Source: CAD feature listing. Evaluate the final solid. Frame: model axes, mm. A direction names the side the tool comes from. Give positions to 0.01 mm unless a question says otherwise; leave off trailing zeros. Loops run counter-clockwise (first coordinate to the right, second up) from the corner with the lowest first, then second, coordinate; pieces in that order, holes last.
from build123d import *

# Parameters (mm, degrees)
SKETCH1_W                   = 65
SKETCH1_H                   = 70
BOSS_EXTRUDE1_DEPTH         = 8
FILLET1_R                   = 5
SKETCH2_W                   = 41
SKETCH2_H                   = 4
BOSS_EXTRUDE2_DEPTH         = 7.87989528
FILLET2_R                   = 2
SKETCH_1_R                  = 1.75
CUT_EXTRUDE_1_DEPTH         = 71
HOLE_WIZARD_M3_1_D          = 2.5
HOLE_WIZARD_M3_1_DEPTH      = 10
HOLE_WIZARD_M3_1_TIP        = 0.751075774
SKETCH_11_W                 = 65
SKETCH_11_H                 = 70.4
EXTRUDE_1_DEPTH             = 2.9
FILLET_2_R                  = 5
FILLET_3_R                  = 5
FILLET_4_R                  = 5
FILLET_5_R                  = 5
SKETCH_24_W                 = 1.25
SKETCH_24_H                 = 2.901
HOLE_WIZARD_M3_2_AT_2_COUNT = 2
HOLE_WIZARD_M3_2_AT_2_PITCH = 50
HOLE_WIZARD_M3_2_AT_3_COUNT = 2
HOLE_WIZARD_M3_2_AT_3_PITCH = 50
HOLE_WIZARD_M3_2_AT_4_COUNT = 2
HOLE_WIZARD_M3_2_AT_4_PITCH = 70.710678119
HOLE_WIZARD_M4_2_AT_2_COUNT = 2
HOLE_WIZARD_M4_2_AT_2_PITCH = 17.145
HOLE_WIZARD_M4_2_AT_3_COUNT = 2
HOLE_WIZARD_M4_2_AT_3_PITCH = 34.29
HOLE_WIZARD_M4_2_AT_4_COUNT = 2
HOLE_WIZARD_M4_2_AT_4_PITCH = 29.696011096
SKETCH_28_W                 = 16.34592277
SKETCH_28_H                 = 84.825432557
CUT_EXTRUDE_4_DEPTH         = 66
HOLE_WIZARD_M6_1_D          = 5


with BuildPart() as part:
    # Sketch1 → Boss-Extrude1 (new body)
    with BuildSketch(Plane.XY):
        Rectangle(SKETCH1_W, SKETCH1_H)
    extrude(amount=BOSS_EXTRUDE1_DEPTH)

    # Fillet1
    fillet1_edges = [part.edges().sort_by_distance(p)[0] for p in [
        (32.5, -35, 4),
        (-32.5, -35, 4),
        (-32.5, 35, 4),
        (32.5, 35, 4),
    ]]
    fillet(fillet1_edges, radius=FILLET1_R)

    # Sketch2 → Boss-Extrude2 (add)
    with BuildSketch(Plane.XY.offset(8)):
        with Locations((0, -33)):
            Rectangle(SKETCH2_W, SKETCH2_H)
    extrude(amount=BOSS_EXTRUDE2_DEPTH)

    # Fillet2
    fillet2_edges = [part.edges().sort_by_distance(p)[0] for p in [
        (-20.5, -33, 8),
        (20.5, -33, 8),
        (-20.5, -33, 15.87989528),
        (20.5, -33, 15.87989528),
    ]]
    fillet(fillet2_edges, radius=FILLET2_R)

    # 草图1 → 切除-拉伸1 (cut, through all)
    with BuildSketch(Plane.XZ.offset(35)):
        with Locations((-16, 11.87989528)):
            Circle(SKETCH_1_R)
        with Locations((0, 11.87989528)):
            Circle(SKETCH_1_R)
        with Locations((16, 11.87989528)):
            Circle(SKETCH_1_R)
    extrude(amount=-CUT_EXTRUDE_1_DEPTH, mode=Mode.SUBTRACT)

    # M3 螺纹孔1
    with Locations(Plane(origin=(25, -19, 0), x_dir=(-1, 0, 0), z_dir=(0, 0, -1))):
        with Locations((0, 0), (0, 50), (50, 50), (50, 0)):
            Hole(HOLE_WIZARD_M3_1_D / 2, depth=HOLE_WIZARD_M3_1_DEPTH)
            with Locations((0, 0, -(HOLE_WIZARD_M3_1_DEPTH + HOLE_WIZARD_M3_1_TIP / 2))):  # 118° drill point
                Cone(0, HOLE_WIZARD_M3_1_D / 2, HOLE_WIZARD_M3_1_TIP, mode=Mode.SUBTRACT)

    # M6 螺纹孔1 (through all)
    with Locations(Plane(origin=(12.3825, 6, 0), x_dir=(-1, 0, 0), z_dir=(0, 0, -1))):
        with Locations((0, 0), (24.765, 0)):
            Hole(HOLE_WIZARD_M6_1_D / 2)


with BuildPart() as body_2:
    # 草图11 → 凸台-拉伸1 (new body)
    with BuildSketch(Plane(origin=(0, 0, -30.31), x_dir=(-1, 0, 0), z_dir=(0, 0, -1))):
        with Locations((0, 0.2)):
            Rectangle(SKETCH_11_W, SKETCH_11_H)
    extrude(amount=-EXTRUDE_1_DEPTH)

    # 圆角2
    fillet_2_edges = [body_2.edges().sort_by_distance(p)[0] for p in [
        (-32.5, 35.4, -28.86),
    ]]
    fillet(fillet_2_edges, radius=FILLET_2_R)

    # 圆角3
    fillet_3_edges = [body_2.edges().sort_by_distance(p)[0] for p in [
        (-32.5, -35, -28.86),
    ]]
    fillet(fillet_3_edges, radius=FILLET_3_R)

    # 圆角4
    fillet_4_edges = [body_2.edges().sort_by_distance(p)[0] for p in [
        (32.5, -35, -28.86),
    ]]
    fillet(fillet_4_edges, radius=FILLET_4_R)

    # 圆角5
    fillet_5_edges = [body_2.edges().sort_by_distance(p)[0] for p in [
        (32.5, 35.4, -28.86),
    ]]
    fillet(fillet_5_edges, radius=FILLET_5_R)

    # 草图24 → M3 螺纹孔2 (revolve, cut)
    with BuildSketch(Plane(origin=(25, 31, -30.31), x_dir=(0, 1, 0), z_dir=(1, 0, 0))):
        with Locations((0.625, 1.4505)):
            Rectangle(SKETCH_24_W, SKETCH_24_H)
    hole_wizard_m3_2 = revolve(axis=Axis((25, 31, -36.66), (0, 0, 1)), mode=Mode.SUBTRACT)

    # M3 螺纹孔2 at 2: M3 螺纹孔2 ×2
    with Locations(*[(-i * HOLE_WIZARD_M3_2_AT_2_PITCH, 0, 0) for i in range(1, HOLE_WIZARD_M3_2_AT_2_COUNT)]):
        add(hole_wizard_m3_2, mode=Mode.SUBTRACT)

    # M3 螺纹孔2 at 3: M3 螺纹孔2 ×2
    with Locations(*[(0, -i * HOLE_WIZARD_M3_2_AT_3_PITCH, 0) for i in range(1, HOLE_WIZARD_M3_2_AT_3_COUNT)]):
        add(hole_wizard_m3_2, mode=Mode.SUBTRACT)

    # M3 螺纹孔2 at 4: M3 螺纹孔2 ×2
    with Locations(*[Vector(-0.707106781, -0.707106781, 0) * (i * HOLE_WIZARD_M3_2_AT_4_PITCH) for i in range(1, HOLE_WIZARD_M3_2_AT_4_COUNT)]):
        add(hole_wizard_m3_2, mode=Mode.SUBTRACT)

    # 草图27 → M4 六角凹头螺钉的柱形沉头孔2 (revolve, cut)
    with BuildSketch(Plane(origin=(9.41775, -9.820005548, -30.31), x_dir=(0, 1, 0), z_dir=(1, 0, 0))):
        Polygon((0, 0), (0, 38.31), (2.25, 38.31), (2.25, 1.5), (4, 1.5), (4, 0), align=None)
    hole_wizard_m4_2 = revolve(axis=Axis((9.41775, -9.820005548, -36.66), (0, 0, 1)), mode=Mode.SUBTRACT)

    # M4 六角凹头螺钉的柱形沉头孔2 at 2: M4 六角凹头螺钉的柱形沉头孔2 ×2
    with Locations(*[(-i * HOLE_WIZARD_M4_2_AT_2_PITCH, 0, 0) for i in range(1, HOLE_WIZARD_M4_2_AT_2_COUNT)]):
        add(hole_wizard_m4_2, mode=Mode.SUBTRACT)

    # M4 六角凹头螺钉的柱形沉头孔2 at 3: M4 六角凹头螺钉的柱形沉头孔2 ×2
    with Locations(*[Vector(-0.5, 0.866025404, 0) * (i * HOLE_WIZARD_M4_2_AT_3_PITCH) for i in range(1, HOLE_WIZARD_M4_2_AT_3_COUNT)]):
        add(hole_wizard_m4_2, mode=Mode.SUBTRACT)

    # M4 六角凹头螺钉的柱形沉头孔2 at 4: M4 六角凹头螺钉的柱形沉头孔2 ×2
    with Locations(*[(0, i * HOLE_WIZARD_M4_2_AT_4_PITCH, 0) for i in range(1, HOLE_WIZARD_M4_2_AT_4_COUNT)]):
        add(hole_wizard_m4_2, mode=Mode.SUBTRACT)

    # 草图28 → 切除-拉伸4 (cut, through all)
    with BuildSketch(Plane(origin=(32.5, 0, 0), x_dir=(0, 0, -1), z_dir=(1, 0, 0))):
        with Locations((29.455626585, -1.857491224)):
            Rectangle(SKETCH_28_W, SKETCH_28_H)
    extrude(amount=-CUT_EXTRUDE_4_DEPTH, mode=Mode.SUBTRACT)


solid = part.part
1) Ray query, probe 1 along X at (y, z) = (5.5, 3); probe 2 along Y at (x, z) = (25, 2); probe 3 along Y at (x, z) = (13.5, 14). Return the intervals inside material, ascending.
Checks:
probe 1: x = -32.5 to -14.83, -9.93 to 9.93, 14.83 to 32.5
probe 2: y = -35 to -20.25, -17.75 to 29.75, 32.25 to 35
probe 3: y = -35 to -31
2) Cut plane C-C (x = 16). Return loops of the section in (y, z).
Checks:
outline: (-35, 0) - (35, 0) - (35, 8) - (-31, 8) - (-31, 10.13) - (-35, 10.13) - close; (-35, 13.63) - (-31, 13.63) - (-31, 15.88) - (-35, 15.88) - close
3) Cut plane D-D (z = 1.5). Return loops of the section in (x, y), and give its area (3 significant figures).
Checks:
outline: (-32.5, -30) arc R5 ccw to (-27.5, -35) - (27.5, -35) arc R5 ccw to (32.5, -30) - (32.5, 30) arc R5 ccw to (27.5, 35) - (-27.5, 35) arc R5 ccw to (-32.5, 30) - close; hole circle Ø2.5 at (-25, -19); hole circle Ø2.5 at (-25, 31); hole circle Ø5 at (-12.38, 6); hole circle Ø5 at (12.38, 6); hole circle Ø2.5 at (25, -19); hole circle Ø2.5 at (25, 31)
area: 4,470 mm2
4) Cut plane A-A (y = -19). Return loops of the section in (x, z).
Checks:
outline: (-32.5, 0) - (-26.25, 0) - (-26.25, 8) - (-32.5, 8) - close; (-23.75, 0) - (23.75, 0) - (23.75, 8) - (-23.75, 8) - close; (26.25, 0) - (32.5, 0) - (32.5, 8) - (26.25, 8) - close
5) Cut plane B-B (x = 25). Return loops of the section in (y, z).
Checks:
outline: (-35, 0) - (-20.25, 0) - (-20.25, 8) - (-35, 8) - close; (-17.75, 0) - (29.75, 0) - (29.75, 8) - (-17.75, 8) - close; (32.25, 0) - (35, 0) - (35, 8) - (32.25, 8) - close
6) Pull-direction query (X, two-part tool) for faces 4 (the flat face through (0, 0, 0)), 5 (the cylindrical face through (26.155, -19.479, 4.056)), 6 (the flat face through (-20.5, -33, 12)); classes: released by +X, released by -X, zero draft, split by the parting line, or undercut.
Checks:
face 4: zero draft
face 5: undercut
face 6: released by -X
7) Reachability of faces 1 (the cylindrical face through (26.155, 30.521, 4.056)), 2 (the flat face through (20.5, -33, 12)), 3 (the flat face through (0, -31, 14)) from +Z, -Z, +X, -X, +Y, -Y: full face, straight path, thin tool, end or side. Return the list, or none.
Checks:
face 1: +Z, -Z
face 2: +Z, +X, +Y, -Y
face 3: +Z, +X, -X, +Y
8) Contact query for flat-ended pins moving along their axis: P1, Ø4.5, axis at y = -34, z = 12, coming from the -X side; P2, Ø3, axis at x = -12.38, y = 6, coming from the -Z side; P3, Ø4, axis at x = 16, z = 11.88, coming from the +Y side; P4, Ø4.5, axis at y = -34, z = 12, coming from the +X side. Output: stop coordinate, or through.
Checks:
P1: stops at x = -20.52
P2: passes through
P3: stops at y = -31
P4: stops at x = 20.52
